Autodesk Inventor part; units mm, degrees
ref_plane "YZ Plane" through (0, 0, 0) normal (1, 0, 0) x (0, 1, 0)
ref_plane "XZ Plane" through (0, 0, 0) normal (0, 1, 0) x (-1, 0, 0)
ref_plane "XY Plane" through (0, 0, 0) normal (0, 0, 1) x (1, 0, 0)
sketch "スケッチ1" plane through (0, 0, 0) normal (0, 1, 0) x (-1, 0, 0)
  line L0 (0, 109.6209) -> (0, -190.3791) construction
  line L1 (-30, 109.6209) -> (-30, -190.3791)
  line L2 (30, -190.3791) -> (30, 109.6209)
  arc A0 (30, 109.6209) -> (-30, 109.6209) centre (0, 109.6209) ccw
  arc A1 (-30, -190.3791) -> (30, -190.3791) centre (0, -190.3791) ccw
  line L3 (0, 109.6209) -> (0, -190.3791) construction
  line L4 (-28.13, 109.6209) -> (-28.13, -190.3791)
  line L5 (28.13, -190.3791) -> (28.13, 109.6209)
  arc A2 (28.13, 109.6209) -> (-28.13, 109.6209) centre (0, 109.6209) ccw
  arc A3 (-28.13, -190.3791) -> (28.13, -190.3791) centre (0, -190.3791) ccw
  point P0 (0, 0)
  point P1 (0, -40.3791)
  point P2 (0, -40.3791)
  dimension "d0" = 300
  dimension "d1" = 60
  dimension "d2" = 56.26
extrude "押し出し1" add sketch "スケッチ1" along normal blind 40
equation "\"BendRadius\" = Thickness"
equation "\"BendReliefWidth\" = Thickness"
equation "\"BendReliefDepth\" = 0.5 * Thickness"
equation "\"CornerReliefSize\" = 4 * Thickness"
equation "\"MinimumRemnant\" = 2 * Thickness"
equation "\"TransitionRadius\" = BendRadius"
equation "\"JacobiRadiusSize\" = BendRadius"
equation "\"GapSize\" = Thickness"
properties part number "0nhk"
Here's how the part is built. I have some questions about the finished solid (model axes, mm). A direction names the side the tool comes from. Round coordinates to 2 decimals unless told otherwise and drop trailing zeros. Write each loop counter-clockwise with the first axis right and the second up, starting at its lowest first coordinate (ties: lowest second). Pieces come first, ordered by that corner, then holes.
1. I need wall thicknesses on L1, parallel to X at y = 7.5, z = -90; L2, parallel to Z at x = 1.5, y = 35; L3, parallel to Z at x = -2, y = 29.5. Which ranges of each line are inside material? Lowest first, please.
2. For faces 5 (the flat face through (29, 0, -40)), 6 (the flat face through (-28.13, 20, -42)), which set-ups out of +Z, -Z, +X, -X, +Y, -Y let a thin tool reach every point of the face, with its end or its side?
3. Suppose I cut it at A-A (x = 0). List the corners of the cut face in (y, z) for me.
4. Suppose I cut it at B-B (z = -92.5). List the corners of the cut face in (x, y) for me, and give its area (3 significant figures).
5. If we mould it in two halves opening along X, with no side actions, what happens to faces 1 (the flat face through (29, 40, -40)), 2 (the cylindrical face through (-0.619, 19.72, -218.502)), 3 (the cylindrical face through (0.66, 19.72, 139.614)), 4 (the flat face through (30, 20, -38))? For each: released by +X, released by -X, zero draft, split by the parting line, or undercut.
6. Will these pins go through, and if not, where does the flat tip stop? pin 1 Ø12 at (x, y) = (-2, 14.5) entering from -Z; pin 2 Ø10 at (x, z) = (-23.5, -65) entering from -Y; pin 3 Ø5 at (x, y) = (8, 5.5) entering from -Z.
7. Suppose I cut it at C-C (y = 6.5). List the corners of the cut face in (x, z) for me.
Answer sheet:
1. L1: x = -30 to -28.13, 28.13 to 30
1. L2: z = -220.34 to -218.47, 137.71 to 139.58
1. L3: z = -220.31 to -218.44, 137.68 to 139.55
2. face 5: +Z, -Z, +X, -X, -Y
2. face 6: +Y, -Y
3. outline: (0, -220.38) - (40, -220.38) - (40, -218.51) - (0, -218.51) - close; (0, 137.75) - (40, 137.75) - (40, 139.62) - (0, 139.62) - close
4. outline: (-30, 0) - (-28.13, 0) - (-28.13, 40) - (-30, 40) - close; (28.13, 0) - (30, 0) - (30, 40) - (28.13, 40) - close
4. area: 150 mm2
5. face 1: zero draft
5. face 2: undercut
5. face 3: split by the parting line
5. face 4: released by +X
6. pin 1: stops at z = -220.38
6. pin 2: stops at y = 0
6. pin 3: stops at z = -219.87
7. outline: (-30, -190.38) arc R30 ccw to (30, -190.38) - (30, 109.62) arc R30 ccw to (-30, 109.62) - close; hole (-28.13, -190.38) arc R28.13 ccw to (28.13, -190.38) - (28.13, 109.62) arc R28.13 ccw to (-28.13, 109.62) - close
